Input: part model. Units: mm. Frame: model coordinates. Face numbers are marked on the shaded views. A direction names the side the tool comes from. Round coordinates to 2 decimals unless told otherwise and drop trailing zeros. Loops run counter-clockwise (first coordinate to the right, second up) from the corner with the lowest first, then second, coordinate; pieces in that order, holes last. Notation, with made-up numbers: (22, -24) -> (32, -24) arc R13 cw to (32, 1) -> close; hole circle Ø5 at (-33.75, 64). An arc over 180 degrees is marked (long way). One line per question, with ' | ' between items. Start each with the question number.
Q1. Cut plane D-D on x = -17.5. Return loops of the section in (y, z).
Q2. Material intervals for L1, parallel to X at y = 12, z = 25; L2, parallel to X at y = -13.5, z = 4.5; L3, parallel to Z at x = 28, y = 8, sorted ascending.
Q3. Contact query for flat-ended pins moving along their axis: P1, Ø5, axis at x = -11, y = 11.5, coming from the -Z side; P2, Ø19, axis at x = 12.5, y = -3, coming from the +Z side; P3, Ø16, axis at x = -12.5, z = 26, coming from the -Y side; P4, Ø10, axis at x = 14.5, z = 12.5, coming from the +Y side. Output: stop coordinate, or through.
Q4. Access query for the marked faces 1, 2, 3, 4 and 5. Directions: +Z, -Z, +X, -X, +Y, -Y. A direction counts if a zero-diameter tool reaches every point of the face in a straight line with its end or side. Return the directions, or none.
Q5. Mould query, pull axis X, two halves, no side actions, for the marked faces 6, 7, 8 and 9. Classes: pulls with the +X half, pulls with the -X half, needs draft (parallel to the pull), parting line crosses it, or undercut.
Q6. Cut plane B-B on y = 9. Return loops of the section in (x, z).
Q7. Cut plane A-A on y = 13.5. Return loops of the section in (x, z), and give its area (3 significant figures).
Q8. Cut plane C-C on z = 22.5. Return loops of the section in (x, y).
from build123d import *

# Parameters (mm, degrees)
F0_W      = 57.15
F0_H      = 38.1
F1_DEPTH  = 6.35
F2_W      = 25.4
F2_H      = 12.7
F3_DEPTH  = 31.75
F4_R      = 6.35
F5_DEPTH  = 25.4
F6_W      = 12.7
F6_H      = 12.7
F7_DEPTH  = 12.7
F9_DEPTH  = 25.4
F10_R     = 3.175
F11_DEPTH = 25.4


with BuildPart() as f1:
    # F0 (on Top) → F1 (new body)
    with BuildSketch(Plane.XY):
        with Locations((3.8689542562, -1.9632895614)):
            Rectangle(F0_W, F0_H)
    extrude(amount=F1_DEPTH)

    # F2 (on face) → F3 (join)
    with BuildSketch(Plane.XY.offset(6.35)):
        with Locations((-12.0060457438, 10.7367104386)):
            Rectangle(F2_W, F2_H)
    extrude(amount=F3_DEPTH)

    # F4 (on face) → F5 (cut)
    with BuildSketch(Plane.XZ.offset(-4.3867104386)):
        with BuildLine():
            ThreePointArc((-24.7060457438, 25.4), (-20.9863018648, 34.380256121), (-12.0060457438, 38.0999999999))
            Line((-12.0060457438, 38.1), (-24.7060457438, 38.1))
            Line((-24.7060457438, 38.1), (-24.7060457438, 25.4))
        make_face()
        with BuildLine():
            ThreePointArc((-12.0060457438, 38.0999999999), (-3.0257896228, 34.3802561209), (0.6939542562, 25.3999999999))
            Line((0.6939542562, 25.3999999999), (0.6939542562, 38.1))
            Line((0.6939542562, 38.1), (-12.0060457438, 38.1))
        make_face()
        with Locations((-12.0060457438, 25.3999999999)):
            Circle(F4_R)
    extrude(amount=-F5_DEPTH, mode=Mode.SUBTRACT)

    # F6 (on face) → F7 (join)
    with BuildSketch(Plane.XY.offset(6.35)):
        with Locations((7.0439542562, 10.7367104386)):
            Rectangle(F6_W, F6_H)
    extrude(amount=F7_DEPTH)

    # F8 (on face) → F9 (cut)
    with BuildSketch(Plane.XZ.offset(-4.3867104386)):
        with BuildLine():
            Line((13.3939542562, 19.05), (0.6939542562, 19.05))
            ThreePointArc((0.6939542562, 19.05), (4.4136981351, 10.0697438789), (13.3939542562, 6.35))
            Line((13.3939542562, 6.35), (13.3939542562, 19.05))
        make_face()
    extrude(amount=-F9_DEPTH, mode=Mode.SUBTRACT)

    # F10 (on face) → F11 (cut)
    with BuildSketch(Plane.XY.offset(6.35)):
        with Locations((-15.1810457438, -11.4882895614)):
            Circle(F10_R)
        with Locations((22.9189542562, -11.4882895614)):
            Circle(F10_R)
        with Locations((22.9189542562, 7.5617104386)):
            Circle(F10_R)
    extrude(amount=-F11_DEPTH, mode=Mode.SUBTRACT)


solid = f1.part
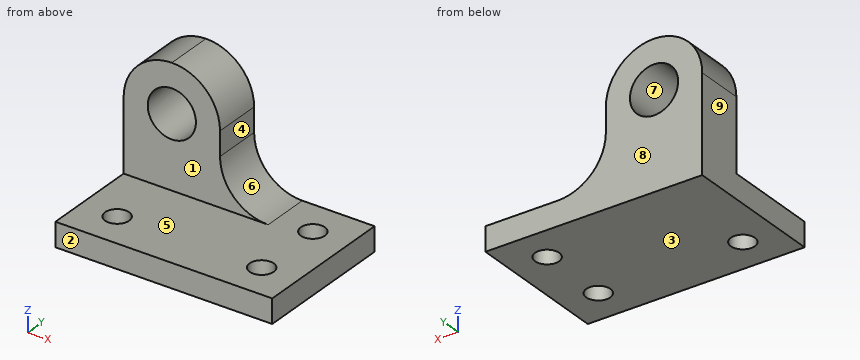
Results:
1) outline: (-21.01, 0) -> (-13.66, 0) -> (-13.66, 6.35) -> (-21.01, 6.35) -> close; (-9.32, 0) -> (17.09, 0) -> (17.09, 22.22) -> (4.39, 22.22) -> (4.39, 6.35) -> (-9.32, 6.35) -> close; (4.39, 28.58) -> (17.09, 28.58) -> (17.09, 36.85) -> (4.39, 36.85) -> close
2) L1: -24.71 to -18.34, -5.67 to 0.69 | L2: -24.71 to -17.64, -12.72 to 20.46, 25.38 to 32.44 | L3: 0 to 6.35
3) P1: z = 0 | P2: z = 8.37 | P3: y = 4.39 | P4: through
4) face 1: +Z, +X, -X, -Y | face 2: +Z, -Z, +X, -X, -Y | face 3: -Z, +X, -X, +Y, -Y | face 4: +Z, +X, +Y, -Y | face 5: +Z, +X, -Y
5) face 6: pulls with the +X half | face 7: undercut | face 8: needs draft | face 9: pulls with the -X half
6) outline: (-24.71, 0) -> (20.09, 0) -> (20.09, 6.35) -> (13.39, 6.35) arc R12.7 cw to (0.69, 19.05) -> (0.69, 25.4) arc R12.7 ccw to (-24.71, 25.4) -> close; (25.75, 0) -> (32.44, 0) -> (32.44, 6.35) -> (25.75, 6.35) -> close; hole circle Ø12.7 at (-12.01, 25.4)
7) outline: (-24.71, 0) -> (32.44, 0) -> (32.44, 6.35) -> (13.39, 6.35) arc R12.7 cw to (0.69, 19.05) -> (0.69, 25.4) arc R12.7 ccw to (-24.71, 25.4) -> close; hole circle Ø12.7 at (-12.01, 25.4) | area: 1,010 mm^2
8) outline: (-24.71, 4.39) -> (-17.66, 4.39) -> (-17.66, 17.09) -> (-24.71, 17.09) -> close; (-6.36, 4.39) -> (0.69, 4.39) -> (0.69, 17.09) -> (-6.36, 17.09) -> close
